from build123d import *

# Parameters (mm, degrees)
SKETCH002_W     = 10
SKETCH002_H     = 46.5
PAD001_DEPTH    = 20
SKETCH003_W     = 10
SKETCH003_H     = 4
POCKET001_DEPTH = 20
SKETCH004_R     = 1.5
POCKET002_DEPTH = 5


with BuildPart() as part:
    # Sketch002 → Pad001 (new body)
    with BuildSketch(Plane.XY):
        Rectangle(SKETCH002_W, SKETCH002_H)
    extrude(amount=PAD001_DEPTH)

    # Sketch003 (on Face6 of Pad001) → Pocket001 (cut)
    with BuildSketch(Plane.XY.offset(20)):
        with Locations((2.5, 20.4)):
            Rectangle(SKETCH003_W, SKETCH003_H)
        with Locations((2.5, 10.2)):
            Rectangle(SKETCH003_W, SKETCH003_H)
        with Locations((2.5, 15.3)):
            Rectangle(SKETCH003_W, SKETCH003_H)
        with Locations((2.5, 5.1)):
            Rectangle(SKETCH003_W, SKETCH003_H)
        with Locations((2.5, 0)):
            Rectangle(SKETCH003_W, SKETCH003_H)
        with Locations((2.5, -20.4)):
            Rectangle(SKETCH003_W, SKETCH003_H)
        with Locations((2.5, -15.3)):
            Rectangle(SKETCH003_W, SKETCH003_H)
        with Locations((2.5, -10.2)):
            Rectangle(SKETCH003_W, SKETCH003_H)
        with Locations((2.5, -5.1)):
            Rectangle(SKETCH003_W, SKETCH003_H)
    extrude(amount=-POCKET001_DEPTH, mode=Mode.SUBTRACT)

    # Sketch004 (on Face26 of Pocket001) → Pocket002 (cut)
    with BuildSketch(Plane.YZ.offset(-2.5)):
        with Locations((0, 15)):
            Circle(SKETCH004_R)
    extrude(amount=-POCKET002_DEPTH, mode=Mode.SUBTRACT)


with BuildPart() as part_1:
    # Body001 placement: moved
    add(part.part.moved(Location((18.5, 0, 1.65))))


solid = part_1.part
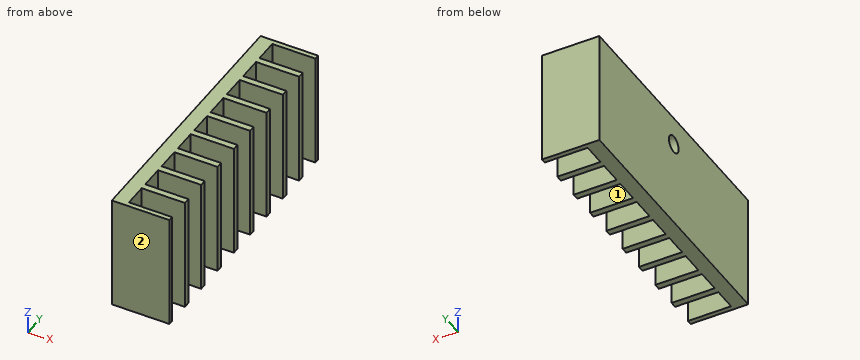
Input: part model. Units: mm. Frame: model coordinates. Face numbers are marked on the shaded views. A direction names the side the tool comes from. Coordinates: 2 decimals unless noted, no trailing zeros. Loops run counter-clockwise (first coordinate to the right, second up) from the corner with the lowest first, then second, coordinate; pieces in that order, holes last.
(1) First-contact query: pin 1 Ø1.2 at (y, z) = (9.5, 10) entering from +X. Flat tip, straight axial feed; report the tip coordinate or a pass-through.
(2) Material intervals for probe 1 along Z at (x, y) = (14.9, 0); probe 2 along X at (y, z) = (-5, 13.75); probe 3 along Y at (x, z) = (14, 17.25), sorted ascending.
(3) Section C-C on y = 14. Return the cut outline in (x, z), then the cut area to 3 significant figures.
(4) Set-up query: the marked faces 1 and 2. Return all of +Z, -Z, +X, -X, +Y, -Y with unobstructed straight access to the full face (end or side cutting, diameter ignored); none if empty.
(5) Section B-B on x = 22. Count the separate pieces of the cut face and the enclosed holes in it, then the cut area to 3 significant figures.
(6) Section A-A on y = 0. Return the cut outline in (x, z), then the cut area to 3 significant figures.
Data:
1. pin 1: stops at x = 16
2. probe 1: z = 1.65 to 15.15, 18.15 to 21.65
2. probe 2: x = 13.5 to 16
2. probe 3: y = -23.25 to -1.37, 1.37 to 23.25
3. outline: (13.5, 1.65) - (16, 1.65) - (16, 21.65) - (13.5, 21.65) - close
3. area: 50.0 mm2
4. face 1: +Z, -Z, +X
4. face 2: +Z, -Z, +X, -X, -Y
5. separate pieces: 10
5. enclosed holes: 0
5. area: 210 mm2
6. outline: (13.5, 1.65) - (16, 1.65) - (16, 15.15) - (13.5, 15.15) - close; (13.5, 18.15) - (16, 18.15) - (16, 21.65) - (13.5, 21.65) - close
6. area: 42.5 mm2
